Read the model definition and answer for the solid it produces. Units are mm, in the model's axes. Face numbers are marked on the shaded views. Give positions to 0.01 mm unless a question says otherwise; leave off trailing zeros. Order: outer loops, then holes, each group sorted by start corner. A loop starts at its lowest first (then second) coordinate and runs counter-clockwise, first axis right, second up. Notation, with made-up numbers: (-38, 22) - (-21, 22) arc R28 cw to (-21, 43) - close; hole circle Ø4 at (26, -28.5). An arc over 180 degrees is marked (long way). Use a Markdown table: item, result. Add a question column.
1. Consider L1, parallel to Z at x = 14.5, y = 0; L2, parallel to Y at x = 0, z = 44; L3, parallel to Y at x = 0, z = 2.75. Determine where each line is inside the solid, lowest interval first.
2. A cutting plane is placed at D-D on x = -14. Determine the outline of the cut face in (y, z).
3. For a pull along Y with two mould halves and no side action, classify the marked faces 1, 2 and 3 as released by +Y, released by -Y, zero draft, split by the parting line, or undercut.
4. Flat-ended cylindrical pins translate along their axes: P1, Ø8, axis at x = 0, y = 0, coming from the -Z side; P2, Ø2, axis at x = 8, y = -17.5, coming from the +Z side; P3, Ø12, axis at y = -18.5, z = 33, coming from the +X side; P4, Ø4, axis at x = 21, z = 15.5, coming from the +Y side. Find the tip coordinate at first contact, or state that the pin passes through.
5. A cutting plane is placed at B-B on x = 0. Determine the outline of the cut face in (y, z).
6. A cutting plane is placed at C-C on z = 11. Determine the outline of the cut face in (x, y), and give its area (3 significant figures).
7. A cutting plane is placed at A-A on y = 0. Determine the outline of the cut face in (x, z), and give its area (3 significant figures).
Autodesk Fusion 360 part; units mm, degrees
sketch "Boceto1" plane through (0, 0, 0) normal (1, 0, 0) x (0, 1, 0)
sketch "Boceto2" plane through (0, 0, 0) normal (0, 0, 1) x (1, 0, 0)
  circle A0 centre (0, 0) radius 30
  circle A1 centre (0, 0) radius 3
  circle A2 centre (0, 0) radius 6.5
  line L0 (0, -30) -> (0.4326, -27.0314) construction
  circle A3 centre (0, 0) radius 27.0348
  dimension "d1" = 60
  dimension "d2" = 6
  dimension "d3" = 13
  dimension "d4" = 3
extrude "Extruir1" add sketch "Boceto2" along normal blind 12 contours A2
extrude "Extruir3" add sketch "Boceto2" along normal blind 25 contours A3
extrude "Extruir4" add sketch "Boceto2" along normal blind 65 contours A0
hole "Agujero1" at (30, 0, 4.6114) direction (-1, 0, 0) diameter 4.234 depth 29 tip angle 180
extrude "Extruir2" [suppressed]
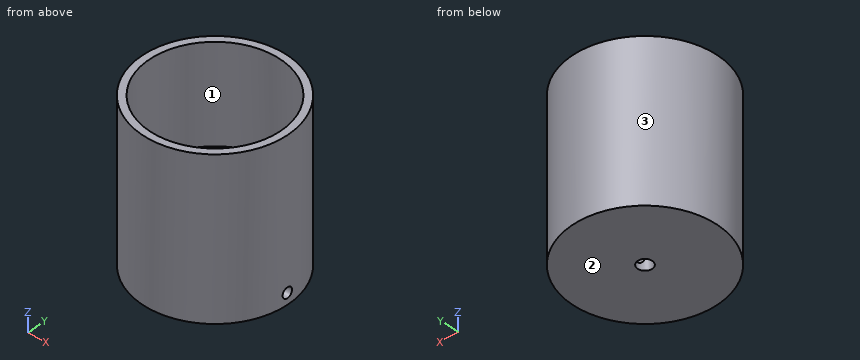
Output values:
| question | item | result |
|---|---|---|
| 1 | L1 | 0 to 2.49, 6.73 to 25 |
| 1 | L2 | -30 to -27.03, 27.03 to 30 |
| 1 | L3 | -30 to -3, 3 to 30 |
| 2 | outline | (-26.53, 0) - (26.53, 0) - (26.53, 65) - (23.13, 65) - (23.13, 25) - (-23.13, 25) - (-23.13, 65) - (-26.53, 65) - close |
| 3 | face 1 | undercut |
| 3 | face 2 | zero draft |
| 3 | face 3 | split by the parting line |
| 4 | P1 | z = 0 |
| 4 | P2 | z = 25 |
| 4 | P3 | x = 27.27 |
| 4 | P4 | y = 23.22 |
| 5 | outline | (-30, 0) - (-3, 0) - (-3, 12) - (-6.5, 12) - (-6.5, 25) - (-27.03, 25) - (-27.03, 65) - (-30, 65) - close; (3, 0) - (30, 0) - (30, 65) - (27.03, 65) - (27.03, 25) - (6.5, 25) - (6.5, 12) - (3, 12) - close |
| 6 | outline | circle Ø60 at (0, 0); hole circle Ø6 at (0, 0) |
| 6 | area | 2,800 mm² |
| 7 | outline | (-30, 0) - (-3, 0) - (-3, 12) - (-6.5, 12) - (-6.5, 25) - (-27.03, 25) - (-27.03, 65) - (-30, 65) - close; (3, 0) - (30, 0) - (30, 2.49) - (3, 2.49) - close; (3, 6.73) - (30, 6.73) - (30, 65) - (27.03, 65) - (27.03, 25) - (6.5, 25) - (6.5, 12) - (3, 12) - close |
| 7 | area | 1,380 mm² |
